Check sheet for the drawn part. Datum: minimum x, y, z corner. Units: mm. Round coordinates to 2 decimals unless told otherwise and drop trailing zeros. Order: outer loops, then holes, each group sorted by start corner. A loop starts at its lowest first (then second) coordinate and runs counter-clockwise, first axis right, second up.
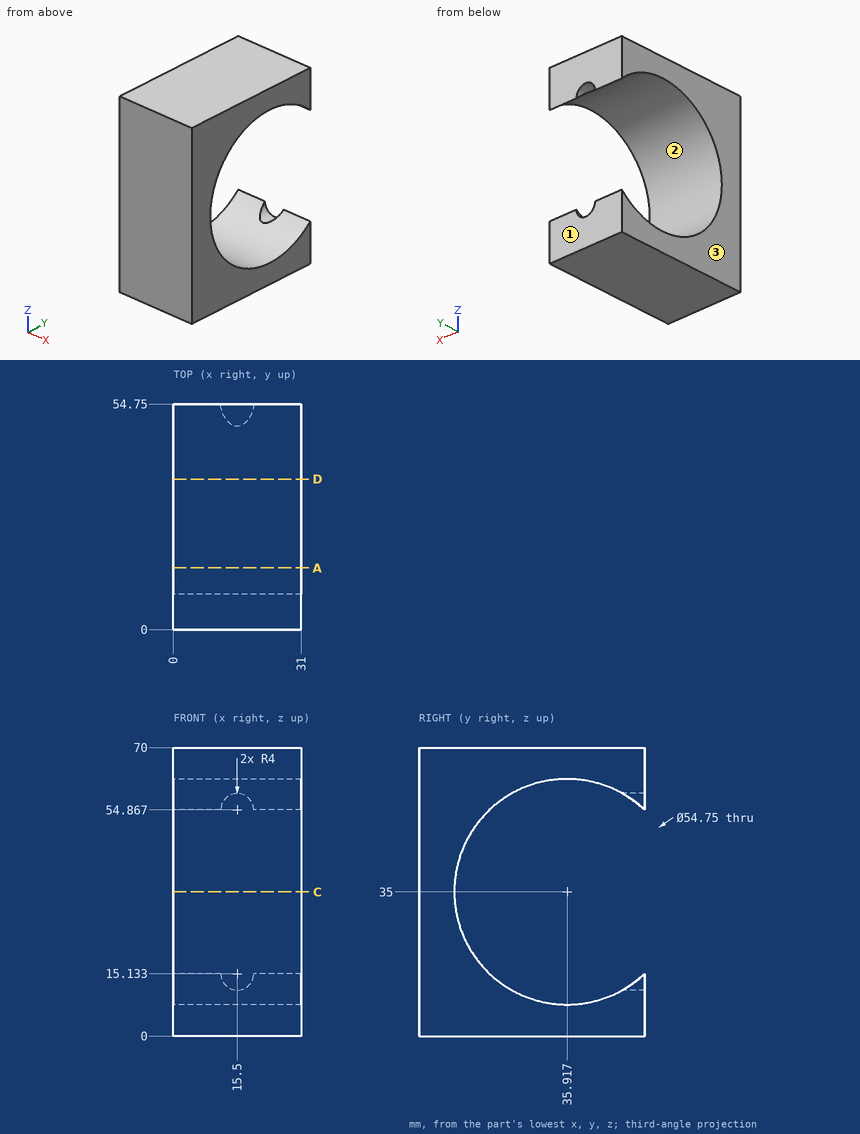
(1) Material ranges on line 1 (Y direction, x = 24, z = 35); line 2 (Z direction, x = 21, y = 33.5); line 3 (Z direction, x = 25, y = 49) (1 decimal), recorded low to high.
Returned:
line 1: y = 0 to 8.54
line 2: z = 0 to 7.73, 62.27 to 70
line 3: z = 0 to 11, 59 to 70
(2) Depth check by flat-ended pin: P1, Ø1.5, axis at x = 6, z = 10, coming from the -Y side; P2, Ø4, axis at x = 27.5, z = 28.5, coming from the +Y side (1 decimal); P3, Ø4, axis at x = 3.5, z = 47, coming from the +Y side. Enter the tip coordinate at first touch or a pass-through.
Returned:
P1: stops at y = 0
P2: stops at y = 9.9
P3: stops at y = 12.39
(3) Sectioned sample at D-D, the plane y = 36.5. Record the cut outline in (x, z).
Returned:
outline: (0, 0) - (31, 0) - (31, 7.63) - (0, 7.63) - close; (0, 62.37) - (31, 62.37) - (31, 70) - (0, 70) - close
(4) Sectioned sample at C-C, the plane z = 35. Record the cut outline in (x, y).
Returned:
outline: (0, 0) - (31, 0) - (31, 8.54) - (0, 8.54) - close
(5) Sectioned sample at A-A, the plane y = 15. Record the cut outline in (x, z).
Returned:
outline: (0, 0) - (31, 0) - (31, 17.34) - (0, 17.34) - close; (0, 52.66) - (31, 52.66) - (31, 70) - (0, 70) - close
(6) Draft check along Y on the marked faces 1, 2 and 3. Enter one of: released by +Y, released by -Y, zero draft, split by the parting line, or undercut.
Returned:
face 1: released by +Y
face 2: undercut
face 3: zero draft
